Geometry: see drawing. Coordinates: mm, zero at the bounding-box minimum. A direction names the side the tool comes from. Round coordinates to 2 decimals unless told otherwise and drop trailing zeros. Order: outer loops, then holes, each group sorted by start corner. A loop starts at its lowest first (then second) coordinate and runs counter-clockwise, first axis right, second up. Notation, with made-up numbers: (-31.5, 37.25) -> (0.5, 37.25) arc R6 ccw to (0.5, 43.25) -> close; hole circle Ø7 at (64.5, -26). An arc over 180 degrees is marked (long way). One line per item, written item: value. Start each with the question number.
1) Section B-B (z = 17). Return the cut outline in (x, y).
2) Section A-A (y = 35). Return the cut outline in (x, z), and give its area (3 significant figures).
3) Section C-C (x = 14). Return the cut outline in (y, z).
4) Pin query (flat end, axial travel): P1, Ø6, axis at x = 41.5, y = 22.5, coming from the -Z side; P2, Ø12, axis at y = 33, z = 104.5, coming from the +X side; P3, Ø10, axis at x = 47.5, y = 6, coming from the +Z side. Return the tip coordinate at first contact, or that it passes through.
5) Ray query, L1, parallel to X at y = 13, z = 43; L2, parallel to Z at x = 31, y = 24. Return the intervals inside material, ascending.
6) Section D-D (y = 45). Return the cut outline in (x, z).
7) Reachability of the marked faces 1, 2 and 3 from +Z, -Z, +X, -X, +Y, -Y: full face, straight path, thin tool, end or side. Return the list, or none.
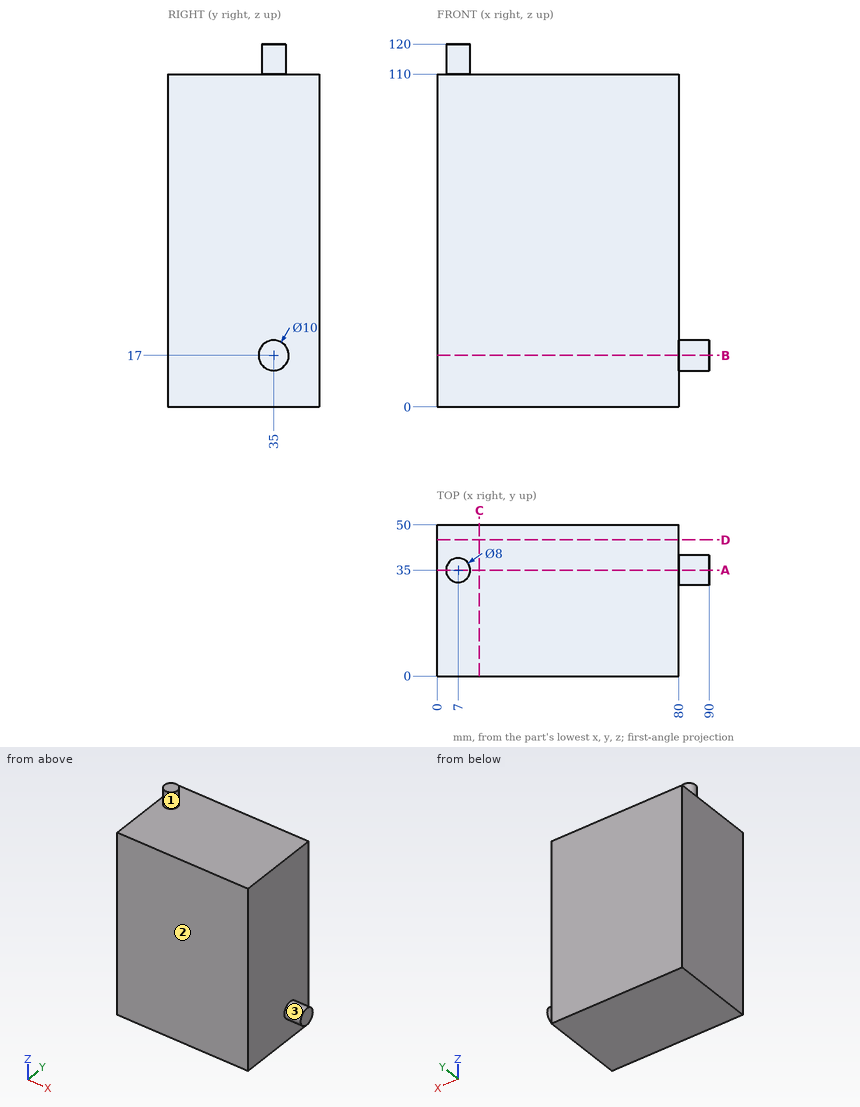
Findings:
1. outline: (0, 0) -> (80, 0) -> (80, 30) -> (90, 30) -> (90, 40) -> (80, 40) -> (80, 50) -> (0, 50) -> close
2. outline: (0, 0) -> (80, 0) -> (80, 12) -> (90, 12) -> (90, 22) -> (80, 22) -> (80, 110) -> (11, 110) -> (11, 120) -> (3, 120) -> (3, 110) -> (0, 110) -> close
2. area: 8,980 mm2
3. outline: (0, 0) -> (50, 0) -> (50, 110) -> (0, 110) -> close
4. P1: z = 0
4. P2: x = 80
4. P3: z = 110
5. L1: 0 to 80
5. L2: 0 to 110
6. outline: (0, 0) -> (80, 0) -> (80, 110) -> (0, 110) -> close
7. face 1: +Z
7. face 2: +Z, -Z, +X, -X, -Y
7. face 3: +X
